Study the drawing (mm; zero at the part's minimum x, y, z) and answer. Round coordinates to 2 decimals unless told otherwise and drop trailing zeros. Order: outer loops, then holes, each group sorted by start corner. A loop starts at its lowest first (then second) coordinate and runs counter-clockwise, first axis right, second up. Notation, with made-up numbers: (32.5, 30) -> (62.5, 30) arc R20 cw to (62.5, 68) -> close; hole circle Ø1 at (43.5, 27). An arc over 180 degrees is marked (long way). Use one line per item in the form item = value.
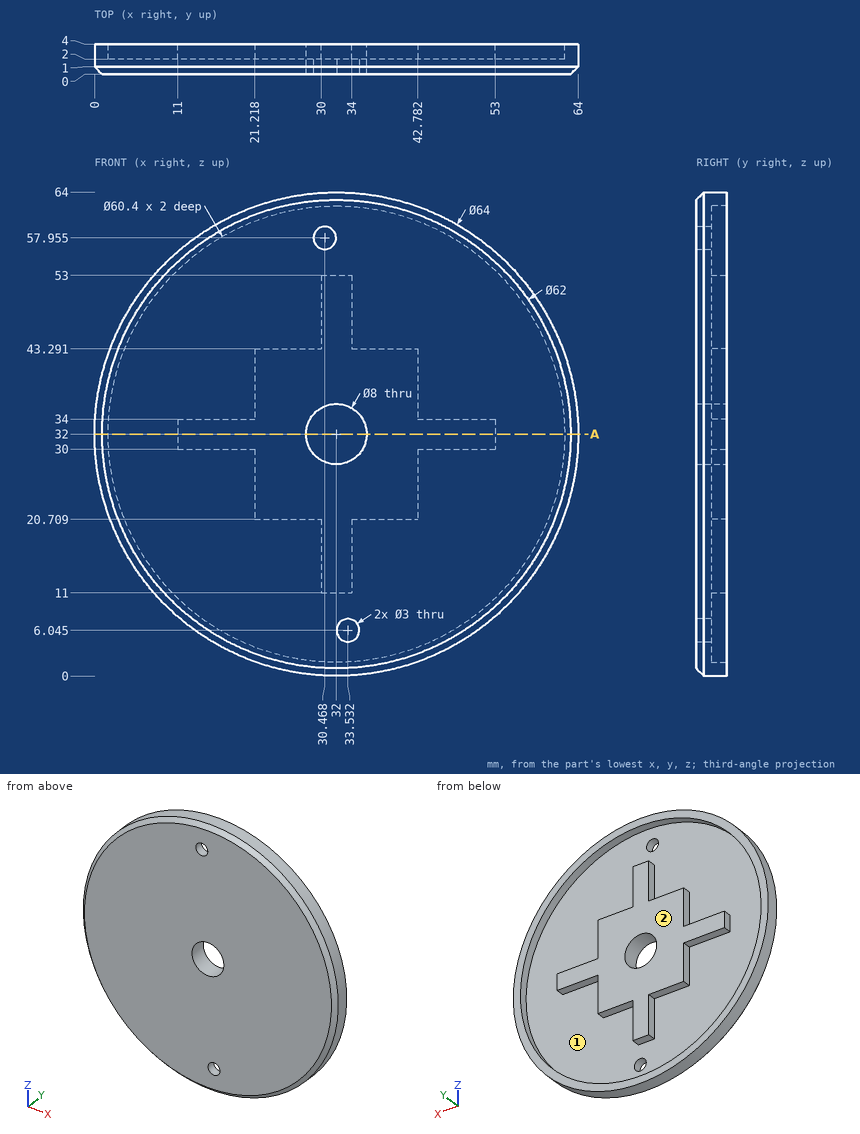
Item 1: Consider line 1 along X through (y, z) = (2.2, 32); line 2 along X through (y, z) = (1.95, 32); line 3 along X through (y, z) = (3.5, 12.5). Determine where each line is inside the solid, lowest interval first.
Findings:
line_1 = 0 to 1.8, 11 to 28, 36 to 53, 62.2 to 64
line_2 = 0 to 28, 36 to 64
line_3 = 6.63 to 8.94, 30 to 34, 55.06 to 57.37
Item 2: The part is cut by section A-A, the plane z = 32. Give the vertices of the cut face in (x, y).
Findings:
outline = (0, 1) -> (1, 0) -> (28, 0) -> (28, 4) -> (11, 4) -> (11, 2) -> (1.8, 2) -> (1.8, 4) -> (0, 4) -> close; (36, 0) -> (63, 0) -> (64, 1) -> (64, 4) -> (62.2, 4) -> (62.2, 2) -> (53, 2) -> (53, 4) -> (36, 4) -> close
Item 3: Determine the mould class of the marked faces 1 and 2 for opening direction Z: released by +Z, released by -Z, zero draft, split by the parting line, or undercut.
Findings:
face_1 = undercut
face_2 = zero draft
Item 4: Flat-ended cylindrical pins translate along their axes: P1, Ø10, axis at x = 14.5, z = 48, coming from the +Y side; P2, Ø2, axis at x = 27.5, y = 3, coming from the -Z side; P3, Ø2, axis at x = 17, y = 3, coming from the +Z side (3 decimals). Find the tip coordinate at first contact, or state that the pin passes through.
Findings:
P1 = 2
P2 = 0.19
P3 = 60.775
